```python
from build123d import *

# Parameters (mm, degrees)
F1_W      = 49
F1_H      = 24
F1_R      = 1.25
F2_DEPTH  = 2
F3_W      = 5
F3_H      = 24
F4_DEPTH  = 4
F5_R      = 1.5
F6_DEPTH  = 24
F7_R      = 2.49999
F8_R      = 3
F9_R      = 8
F10_DEPTH = 2


# Not quite as in the source:
# - a fillet or chamfer is up to 0.001 mm smaller than in the source, because OpenCascade refuses the exact size


with BuildPart() as f2:
    # F1 (on Top) → F2 (new body)
    with BuildSketch(Plane.XY):
        with Locations((-22.5, 10)):
            Rectangle(F1_W, F1_H)
        with Locations((-43, 2)):
            Circle(F1_R, mode=Mode.SUBTRACT)
        with Locations((-2, 2)):
            Circle(F1_R, mode=Mode.SUBTRACT)
        with Locations((-43, 18)):
            Circle(F1_R, mode=Mode.SUBTRACT)
        with Locations((-2, 18)):
            Circle(F1_R, mode=Mode.SUBTRACT)
    extrude(amount=F2_DEPTH)

    # F3 (on face) → F4 (join)
    with BuildSketch(Plane.XY.offset(2)):
        with Locations((-22.5, 10)):
            Rectangle(F3_W, F3_H)
    extrude(amount=F4_DEPTH)

    # F5 (on face) → F6 (cut, through all)
    with BuildSketch(Plane.XZ.offset(2)):
        with Locations((-22.5, 3.5)):
            Circle(F5_R)
    extrude(amount=-F6_DEPTH, mode=Mode.SUBTRACT)

    # F7 (radius 2.5 in the source; OpenCascade refuses exactly that, so slightly less here)
    f7_edges = [f2.edges().sort_by_distance(p)[0] for p in [
        (-20, 10, 6),
        (-25, 10, 6),
    ]]
    fillet(f7_edges, radius=F7_R)

    # F8
    f8_edges = [f2.edges().sort_by_distance(p)[0] for p in [
        (2, -2, 1),
        (2, 22, 1),
        (-47, 22, 1),
        (-47, -2, 1),
    ]]
    fillet(f8_edges, radius=F8_R)

    # F9 (on face) → F10 (cut, through all)
    with BuildSketch(Plane.XY.offset(2)):
        with Locations((-35, 10)):
            Circle(F9_R)
        with Locations((-10, 10)):
            Circle(F9_R)
    extrude(amount=-F10_DEPTH, mode=Mode.SUBTRACT)


solid = f2.part
```
Design review of the part built by this model. Coordinates are the model's own, in mm. A direction names the side the tool comes from. Round coordinates to 2 decimals unless told otherwise and drop trailing zeros. Order: outer loops, then holes, each group sorted by start corner. A loop starts at its lowest first (then second) coordinate and runs counter-clockwise, first axis right, second up. Notation, with made-up numbers: M 21.5,4.25 L 28.5,4.25 A16 ccw 28.5,16.25 Z; hole C 13,49.5 d8. An arc over 180 degrees is marked long. Put each result on its own line as item: value.
Q1. To check wall thickness, follow line 1 (X direction, y = 15, z = 0.85) (3 decimals); line 2 (Y direction, x = -10, z = 0.65); line 3 (X direction, y = 16, z = 1.8). State the ranges of each line that lie inside material, in increasing order.
Reported:
line 1: -47 to -41.245, -28.755 to -16.245, -3.755 to 2
line 2: -2 to 2, 18 to 22
line 3: -47 to -40.29, -29.71 to -15.29, -4.71 to 2
Q2. Draft analysis for pull direction Z (two halves, no side actions). For faces 1 (the face through (-23, 10, 0)), 2 (the face through (-24, 9.83, 3.57)), 3 (the face through (-41.349, 5.132, 1.014)), 4 (the face through (-1.8, 10.2, 2)), state which applies: released by +Z, released by -Z, zero draft, split by the parting line, or undercut.
Reported:
face 1: released by -Z
face 2: undercut
face 3: zero draft
face 4: released by +Z
Q3. Machinability: for faces 5 (the face through (-25, 10, 3)), 6 (the face through (-23, 22, 1)), which of the approach directions +Z, -Z, +X, -X, +Y, -Y give a long, thin tool a straight path to every point of the face, cutting with its end or side? Answer none if there is none.
Reported:
face 5: +Z, -X, +Y, -Y
face 6: +Z, -Z, +X, -X, +Y
Q4. Consider section B-B (x = -35). State the section outline as (y, z) points.
Reported:
outline: M -2,0 L 2,0 L 2,2 L -2,2 Z; M 18,0 L 22,0 L 22,2 L 18,2 Z
Q5. Consider section C-C (z = 1.3). State the section outline as (x, y) points.
Reported:
outline: M -47,1 A3 ccw -44,-2 L -1,-2 A3 ccw 2,1 L 2,19 A3 ccw -1,22 L -44,22 A3 ccw -47,19 Z; hole C -43,2 d2.5; hole C -43,18 d2.5; hole C -35,10 d16; hole C -10,10 d16; hole C -2,2 d2.5; hole C -2,18 d2.5
Q6. Consider section A-A (y = 8.5). State how many separate pieces and enclosed holes the cut face has, and give its area (3 significant figures).
Reported:
separate pieces: 3
enclosed holes: 1
area: 45.4 mm²
Q7. Insertion check: pin 1 Ø11 at (x, y) = (-9.5, 5.5) entering from +Z; pin 2 Ø1.2 at (y, z) = (9.5, 3) entering from -X. Each pin has a flat end and moves straight along its axis. Give the tip position at first contact, or say it passes through.
Reported:
pin 1: z = 2
pin 2: x = -25
